Autodesk Inventor part; units mm, degrees
ref_plane "YZ Plane" through (0, 0, 0) normal (1, 0, 0) x (0, 1, 0)
ref_plane "XZ Plane" through (0, 0, 0) normal (0, 1, 0) x (-1, 0, 0)
ref_plane "XY Plane" through (0, 0, 0) normal (0, 0, 1) x (1, 0, 0)
sketch "草图1" plane through (0, 0, 0) normal (0, 1, 0) x (-1, 0, 0)
  line L0 (-27, 15) -> (7, 15)
  line L1 (27, 0) -> (27, -15)
  line L2 (27, -15) -> (-27, -15)
  line L3 (-27, -15) -> (-27, 15)
  line L4 (-27, 15) -> (27, -15) construction
  line L5 (27, 15) -> (-27, -15) construction
  line L6 (27, 0) -> (7, 15)
  circle A0 centre (17, -5) radius 4
  circle A1 centre (-3, 5) radius 5
  point P0 (0, 0)
  dimension "d0" = 54
  dimension "d1" = 30
  dimension "d2" = 20
  dimension "d3" = 8
  dimension "d4" = 10
  dimension "d5" = 10
  dimension "d6" = 10
  dimension "d7" = 20
  dimension "d8" = 30
extrude "拉伸1" add sketch "草图1" along normal blind 15
sketch "草图2" plane through (0, 0, 0) normal (0, 1, 0) x (-1, 0, 0)
  circle A0 centre (-3, 5) radius 5
  circle A1 centre (17, -5) radius 4
  line L0 (7, 15) -> (-27, 15)
  line L1 (-27, 15) -> (-27, -15)
  line L2 (-27, -15) -> (27, -15)
  line L3 (27, -15) -> (27, 0)
  line L4 (27, 0) -> (7, 15)
  circle A2 centre (-3, 5) radius 7.5
  point P0 (0, 0)
  dimension "d11" = 15
extrude "拉伸2" cut sketch "草图2" along normal blind 6 contours A2
sketch "草图3" plane through (0, 15, 0) normal (0, 1, 0) x (1, 0, 0)
  line L0 (-7, -15) -> (27, -15)
  line L1 (27, -15) -> (27, 15)
  line L2 (27, 15) -> (-27, 15)
  line L3 (17, 15) -> (17, -15)
  point P0 (0, 0)
  dimension "d14" = 10
extrude "拉伸3" add sketch "草图3" along normal blind 8
hole "孔1" at (22, 23, 10) direction (0, -1, 0) diameter 4 depth 12 tip angle 118
hole "孔2" at (22, 23, -10) direction (0, -1, 0) diameter 4 depth 12 tip angle 118
Here's how the part is built. I have some questions about the finished solid (model axes, mm). A direction names the side the tool comes from. Coordinates: 2 decimals unless noted, no trailing zeros. Order: outer loops, then holes, each group sorted by start corner. A loop starts at its lowest first (then second) coordinate and runs counter-clockwise, first axis right, second up. Notation, with made-up numbers: (60.5, 8) - (90.5, 8) arc R24 cw to (90.5, 26) - close; hole circle Ø11 at (49.25, 68). An arc over 180 degrees is marked (long way). One line per question, with ' | ' between items.
(1) Suppose I cut it at D-D on x = 3. List the corners of the cut face in (y, z) for me.
Report:
outline: (0, -15) - (15, -15) - (15, 0) - (6, 0) - (6, -2.5) - (0, -2.5) - close; (0, 12.5) - (6, 12.5) - (6, 10) - (15, 10) - (15, 15) - (0, 15) - close
(2) Will these pins go through, and if not, where does the flat tip stop? pin 1 (5 mm diameter, centred on x = 22, z = 10, fed in from -Y); pin 2 (9 mm diameter, centred on x = -12.5, z = -6, fed in from +Y); pin 3 (4 mm diameter, centred on y = 19.5, z = -5, fed in from -X); pin 4 (5 mm diameter, centred on x = -17, z = -5, fed in from -Y).
Report:
pin 1: stops at y = 0 | pin 2: stops at y = 15 | pin 3: stops at x = 17 | pin 4: passes through
(3) For faces 5 (the flat face through (0, 15, 0)), 6 (the flat face through (-2, 6, 3)), 7 (the cylindrical face through (-13.8, 7.4, -2.6)), 8 (the cylindrical face through (20, 17, -10)), 9 (the flat face through (0, 0, -3)), which set-ups out of +Z, -Z, +X, -X, +Y, -Y let a thin tool reach every point of the face, with its end or its side?
Report:
face 5: +Z, -Z, -X, +Y | face 6: -Y | face 7: +Y, -Y | face 8: +Y | face 9: +Z, -Z, +X, -X, -Y
(4) Suppose I cut it at A-A on x = -17. List the corners of the cut face in (y, z) for me, and give its area (4 significant figures).
Report:
outline: (0, -15) - (15, -15) - (15, -9) - (0, -9) - close; (0, -1) - (15, -1) - (15, 7.5) - (0, 7.5) - close | area: 217.5 mm2
(5) Suppose I cut it at B-B on z = -5. List the corners of the cut face in (x, y) for me.
Report:
outline: (-27, 0) - (-21, 0) - (-21, 15) - (-27, 15) - close; (-13, 0) - (27, 0) - (27, 23) - (17, 23) - (17, 15) - (-13, 15) - close
(6) If we mould it in two halves opening along X, with no side actions, what happens to faces 1 (the flat face through (10, 9, 15)), 2 (the flat face through (-27, 7, -7)), 3 (the conical face through (22.235, 10.007, -10.256)), 4 (the flat face through (27, 11, 0))? For each: pulls with the +X half, pulls with the -X half, needs draft (parallel to the pull), parting line crosses it, or undercut.
Report:
face 1: needs draft | face 2: pulls with the -X half | face 3: undercut | face 4: pulls with the +X half
(7) If I drill on L1, parallel to Z at x = 22, y = 13.75; L2, parallel to X at y = 16, z = -10; L3, parallel to Y at x = -23.5, z = -2.75, over which ranges is the centre line in solid material (lowest first)?
Report:
L1: z = -15 to -12, -8 to 8, 12 to 15 | L2: x = 17 to 20, 24 to 27 | L3: y = 0 to 15
(8) Suppose I cut it at C-C on y = 3.5. List the corners of the cut face in (x, z) for me.
Report:
outline: (-27, -15) - (27, -15) - (27, 15) - (-7, 15) - (-27, 0) - close; hole circle Ø8 at (-17, -5); hole circle Ø15 at (3, 5)
